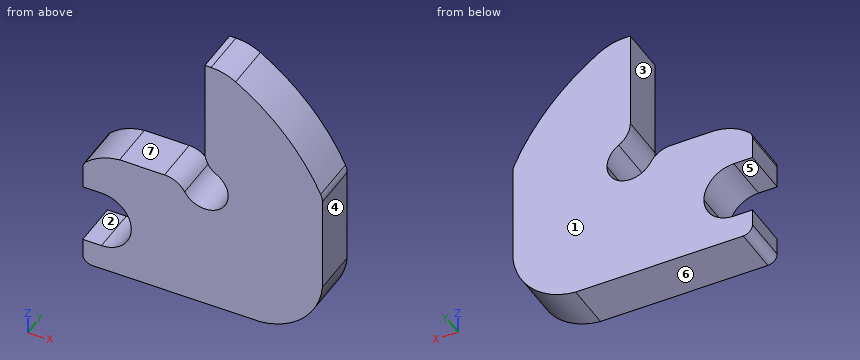
```python
from build123d import *

# Parameters (mm, degrees)
F1_DEPTH = 25
F2_R     = 12.5
F3_R     = 12.5
F4_R     = 25
F5_R     = 5
F6_R     = 5
F7_R     = 10


with BuildPart() as f1:
    # F0 (on Front) → F1 (new body)
    with BuildSketch(Plane.XZ):
        with BuildLine():
            Line((25.221193, 0), (19.72456, 0))
            ThreePointArc((19.72456, 0), (8.907216, -3.116178), (0, -10))
            Line((0, -10), (0, -24))
            Line((0, -24), (10, -24))
            ThreePointArc((10, -24), (21.313708, -28.686292), (26, -40))
            ThreePointArc((26, -40), (21.313708, -51.313708), (10, -56))
            Line((10, -56), (0, -56))
            Line((0, -56), (0, -70))
            Line((0, -70), (88.427416, -70))
            Line((88.427416, -70), (94.69316, -70))
            ThreePointArc((94.69316, -70), (117.723239, -59.295823), (128.427416, -36.265744))
            Line((128.427416, -36.265744), (128.427416, -30))
            Line((128.427416, -30), (128.427416, 18))
            ThreePointArc((128.427416, 18), (106.677114, 50.916386), (75.427416, 75))
            Line((75.427416, 75), (65.427416, 75))
            Line((65.427416, 75), (65.427416, 12.5))
            ThreePointArc((65.427416, 12.5), (74.266251, 8.838835), (77.927416, 0))
            ThreePointArc((77.927416, 0), (65.427416, -12.5), (52.927416, 0))
            Line((52.927416, 0), (25.221193, 0))
        make_face()
    extrude(amount=F1_DEPTH)

    # F2
    f2_edges = [f1.edges().sort_by_distance(p)[0] for p in [
        (65.427416, -12.5, 12.5),
    ]]
    fillet(f2_edges, radius=F2_R)

    # F3
    f3_edges = [f1.edges().sort_by_distance(p)[0] for p in [
        (52.927416, -12.5, 0),
    ]]
    fillet(f3_edges, radius=F3_R)

    # F4
    f4_edges = [f1.edges().sort_by_distance(p)[0] for p in [
        (75.427416, -12.5, 75),
    ]]
    fillet(f4_edges, radius=F4_R)

    # F5
    f5_edges = [f1.edges().sort_by_distance(p)[0] for p in [
        (0, -12.5, -10),
    ]]
    fillet(f5_edges, radius=F5_R)

    # F6
    f6_edges = [f1.edges().sort_by_distance(p)[0] for p in [
        (0, -12.5, -70),
    ]]
    fillet(f6_edges, radius=F6_R)

    # F7
    f7_edges = [f1.edges().sort_by_distance(p)[0] for p in [
        (128.427416, -12.5, 18),
    ]]
    fillet(f7_edges, radius=F7_R)


solid = f1.part
```
Work out the finished part from the listing and answer in its coordinate system (mm). Face numbers are marked on the shaded views. A direction names the side the tool comes from. Round coordinates to 2 decimals unless told otherwise and drop trailing zeros. Write each loop counter-clockwise with the first axis right and the second up, starting at its lowest first coordinate (ties: lowest second). Pieces come first, ordered by that corner, then holes. Notation, with made-up numbers: (27.5, 23.5) - (46.5, 23.5) arc R34 cw to (46.5, 59.5) - close; hole circle Ø4 at (-30, 68). An arc over 180 degrees is marked (long way). Return JSON: item names as keys, results as strings. Group by question number.
Q1. The part is cut by section B-B on x = 75. Write down the section's boundary in (y, z), then the cut area to 3 significant figures.
Q2. For the marked faces 1, 2 and 3, determine the directions among +Z, -Z, +X, -X, +Y, -Y from which every point of the face is accessible in a straight line to the end or side of a thin tool.
Q3. Each of these flat-tipped pins is pushed along its axis until it touches: pin 1 Ø4 at (y, z) = (-5, 40.5) entering from +X; pin 2 Ø1 at (y, z) = (-11.5, -38.5) entering from -X; pin 3 Ø8 at (x, y) = (2.5, -7) entering from +Z. Where does it stop, or does it pass through?
Q4. The part is cut by section A-A on y = -4.75. Write down the section's boundary in (x, z).
Q5. The part is cut by section D-D on x = 35. Write down the section's boundary in (y, z).
Q6. Find the intervals of material crossed by L1, parallel to Z at x = 37, y = -1.75; L2, parallel to X at y = -1.5, z = -9; L3, parallel to Z at x = 13.5, y = -19.75, in increasing order.
Q7. The part is cut by section C-C on z = 49. Write down the section's boundary in (x, y), then the cut area to 3 significant figures.
Q8. The mould has two halves that part along Z. Classify the marked faces 4, 5, 6 and 7: released by +Z, released by -Z, zero draft, split by the parting line, or undercut.
Solved:
{
 "1": {"outline": "(-25, -70) - (0, -70) - (0, -8.04) - (-25, -8.04) - close; (-25, 8.04) - (0, 8.04) - (0, 74.21) - (-25, 74.21) - close", "area": "3,200 mm²"},
 "2": {"face 1": "+Z, -Z, +X, -X, +Y", "face 2": "-X, +Y, -Y", "face 3": "+Z, -X, +Y, -Y"},
 "3": {"pin 1": "x = 116.77", "pin 2": "x = 25.87", "pin 3": "z = -4.48"},
 "4": {"outline": "(0, -65) arc R5 ccw to (5, -70) - (94.69, -70) arc R37 ccw to (128.43, -36.27) - (128.43, 15.83) arc R10 ccw to (127.48, 20.07) arc R120 ccw to (81.92, 71.26) arc R25 ccw to (68.77, 75) - (65.43, 75) - (65.43, 21.65) arc R12.5 ccw to (71.68, 10.83) arc R12.5 cw (long way) to (54.6, -6.25) arc R12.5 ccw to (43.78, 0) - (19.72, 0) arc R30 ccw to (1.51, -8.42) arc R5 ccw to (0, -11.99) - (0, -24) - (10, -24) arc R16 cw to (26, -40) arc R16 cw to (10, -56) - (0, -56) - close"},
 "5": {"outline": "(-25, -70) - (0, -70) - (0, 0) - (-25, 0) - close"},
 "6": {"L1": "-70 to 0", "L2": "1 to 56.75, 74.1 to 128.43", "L3": "-70 to -55.61, -24.39 to -1.25"},
 "7": {"outline": "(65.43, -25) - (108.42, -25) - (108.42, 0) - (65.43, 0) - close", "area": "1,070 mm²"},
 "8": {"face 4": "zero draft", "face 5": "undercut", "face 6": "released by -Z", "face 7": "released by +Z"}
}
